```python
from build123d import *

# Parameters (mm, degrees)
F0_W     = 35.56
F0_H     = 35.56
F1_DEPTH = 5.08
F2_W     = 19.812
F2_H     = 4.572
F3_DEPTH = 2.54
F4_W     = 19.812
F4_H     = 4.572
F5_DEPTH = 2.54
F6_W     = 20.32
F6_H     = 5.08
F7_DEPTH = 2.54
F8_W     = 20.32
F8_H     = 5.08
F9_DEPTH = 2.54


with BuildPart() as f1:
    # F0 (on Top) → F1 (new body, symmetric)
    with BuildSketch(Plane.XY):
        Rectangle(F0_W, F0_H)
        with BuildLine():
            add(Edge.make_bspline(
                [(7.4772352431, 9.2300998264), (10.8892578125, 5.9751736111), (10.8892578125, 0.1322916667)],
                knots=[0, 0, 0, 1, 1, 1], degree=2))
            add(Edge.make_bspline(
                [(10.8892578125, 0.1322916667), (10.8892578125, -6.0854166667), (7.3476996528, -9.3927083333)],
                knots=[0, 0, 0, 1, 1, 1], degree=2))
            add(Edge.make_bspline(
                [(7.3476996528, -9.3927083333), (3.8061414931, -12.7), (-2.8745876736, -12.7)],
                knots=[0, 0, 0, 1, 1, 1], degree=2))
            Line((-2.8745876736, -12.7), (-10.0073133681, -12.7))
            Line((-10.0073133681, -12.7), (-10.0073133681, 12.4850260417))
            Line((-10.0073133681, 12.4850260417), (-2.1028862847, 12.4850260417))
            add(Edge.make_bspline(
                [(-2.1028862847, 12.4850260417), (4.0652126736, 12.4850260417), (7.4772352431, 9.2300998264)],
                knots=[0, 0, 0, 1, 1, 1], degree=2))
        make_face(mode=Mode.SUBTRACT)
    extrude(amount=F1_DEPTH, both=True)

    # F2 (on face) → F3 (join)
    with BuildSketch(Plane(origin=(0, 17.78, 0), x_dir=(-1, 0, 0), z_dir=(0, 1, 0))):
        Rectangle(F2_W, F2_H)
    extrude(amount=F3_DEPTH)

    # F4 (on face) → F5 (join)
    with BuildSketch(Plane(origin=(-17.78, 0, 0), x_dir=(0, -1, 0), z_dir=(-1, 0, 0))):
        Rectangle(F4_W, F4_H)
    extrude(amount=F5_DEPTH)

    # F6 (on face) → F7 (cut)
    with BuildSketch(Plane.XZ.offset(17.78)):
        Rectangle(F6_W, F6_H)
    extrude(amount=-F7_DEPTH, mode=Mode.SUBTRACT)

    # F8 (on face) → F9 (cut)
    with BuildSketch(Plane.YZ.offset(17.78)):
        Rectangle(F8_W, F8_H)
    extrude(amount=-F9_DEPTH, mode=Mode.SUBTRACT)


solid = f1.part
```
Design review of the part built by this model. Coordinates are the model's own, in mm. A direction names the side the tool comes from. Give positions to 0.01 mm unless a question says otherwise; leave off trailing zeros. Order: outer loops, then holes, each group sorted by start corner. A loop starts at its lowest first (then second) coordinate and runs counter-clockwise, first axis right, second up. Notation, with made-up numbers: M 37,-2.75 L 81,-2.75 A22 cw 81,20.25 Z; hole C -34,-21.5 d9. An arc over 180 degrees is marked long. One line per question, with ' | ' between items. Start each with the question number.
Q1. Machinability: for faces 5 (the face through (0, 19, -2.286)), 6 (the face through (-19, 0, -2.286)), 7 (the face through (17, 0, 2.54)), 8 (the face through (9.906, 19, 0)), 9 (the face through (-19, 9.906, 0)), which of the approach directions +Z, -Z, +X, -X, +Y, -Y give a long, thin tool a straight path to every point of the face, cutting with its end or side? Answer none if there is none.
Q2. For pin 1 Ø0.8 at (x, y) = (0.5, 19) entering from +Z; pin 2 Ø1.3 at (y, z) = (19, 0) entering from -X; pin 3 Ø0.8 at (y, z) = (19, 0.5) entering from +X; pin 4 Ø6 at (x, y) = (-6, -0.5) entering from -Z, all flat-tipped, find the tip position at first contact; note any pin that passes through.
Q3. We need section B-B (y = 14.5). Write out the cut boundary in (x, z), plus the area to 3 significant figures.
Q4. The part is to be moulded in two halves that separate along Z. For faces 1 (the face through (-10.007, 0, 0)), 2 (the face through (12, 0, -5.08)), 3 (the face through (17, 0, -2.54)), 4 (the face through (-10.16, -17, 0)), say which applies: +Z half, -Z half, draft (parallel to the pull), parting line (faces both ways), or undercut.
Q5. For L1, parallel to Y at x = -5.5, z = -0.5; L2, parallel to X at y = -15.5, z = -0.25; L3, parallel to Y at x = 14.5, z = 0, list the stretches that pass through material, from the lowest coordinate up. Write a range as [from, to].
Q6. We need section A-A (x = -6.5). Write out the cut boundary in (y, z), plus the area to 3 significant figures.
Returned:
1) face 5: -Z, +X, -X, +Y | face 6: -Z, -X, +Y, -Y | face 7: +X | face 8: +Z, -Z, +X, +Y | face 9: +Z, -Z, -X, +Y
2) pin 1: z = 2.29 | pin 2: x = -9.91 | pin 3: x = 9.91 | pin 4: through
3) outline: M -17.78,-5.08 L 17.78,-5.08 L 17.78,5.08 L -17.78,5.08 Z | area: 361 mm2
4) face 1: draft | face 2: -Z half | face 3: undercut | face 4: undercut
5) L1: [-15.24, -12.7], [12.49, 20.32] | L2: [-17.78, -10.16], [10.16, 17.78] | L3: [-17.78, 17.78]
6) outline: M -17.78,-5.08 L -12.7,-5.08 L -12.7,5.08 L -17.78,5.08 L -17.78,2.54 L -15.24,2.54 L -15.24,-2.54 L -17.78,-2.54 Z; M 12.49,-5.08 L 17.78,-5.08 L 17.78,-2.29 L 20.32,-2.29 L 20.32,2.29 L 17.78,2.29 L 17.78,5.08 L 12.49,5.08 Z | area: 104 mm2
